from build123d import *

# Parameters (mm, degrees)
F0_W     = 106
F0_H     = 100
F0_R     = 2.706104
F0_R_2   = 5
F0_W_2   = 80
F0_H_2   = 52
F1_DEPTH = 31
F2_R     = 10
F3_DEPTH = 2.5
F4_W     = 48
F4_H     = 15
F5_DEPTH = 2.5
F6_W     = 4.25
F6_H     = 28.5
F7_DEPTH = 2.5


with BuildPart() as f1:
    # F0 (on Front) → F1 (new body)
    with BuildSketch(Plane.XZ):
        Rectangle(F0_W, F0_H)
        with Locations((0, -37.5)):
            Circle(F0_R, mode=Mode.SUBTRACT)
        with Locations((16.9, -34.7)):
            Circle(F0_R_2, mode=Mode.SUBTRACT)
        with Locations((32.5, -37.5)):
            Circle(F0_R, mode=Mode.SUBTRACT)
        with Locations((0, 10.5)):
            Rectangle(F0_W_2, F0_H_2, mode=Mode.SUBTRACT)
        with Locations((0, 10.5)):
            Rectangle(F0_W_2, F0_H_2)
        with Locations((0, -37.5)):
            Circle(F0_R)
        with Locations((16.9, -34.7)):
            Circle(F0_R_2)
        with Locations((32.5, -37.5)):
            Circle(F0_R)
    extrude(amount=-F1_DEPTH)

    # F2
    f2_edges = [f1.edges().sort_by_distance(p)[0] for p in [
        (53, 15.5, -50),
        (53, 15.5, 50),
        (-53, 15.5, 50),
        (-53, 15.5, -50),
    ]]
    fillet(f2_edges, radius=F2_R)

    # F0 (on Front) → F3 (cut)
    with BuildSketch(Plane.XZ):
        with Locations((0, 10.5)):
            Rectangle(F0_W_2, F0_H_2)
        with Locations((0, -37.5)):
            Circle(F0_R)
        with Locations((16.9, -34.7)):
            Circle(F0_R_2)
        with Locations((32.5, -37.5)):
            Circle(F0_R)
    extrude(amount=-F3_DEPTH, mode=Mode.SUBTRACT)

    # F4 (on face) → F5 (cut)
    with BuildSketch(Plane(origin=(0, 31, 0), x_dir=(-1, 0, 0), z_dir=(0, 1, 0))):
        with Locations((19, 10)):
            Rectangle(F4_W, F4_H)
    extrude(amount=-F5_DEPTH, mode=Mode.SUBTRACT)

    # F6 (on face) → F7 (cut)
    with BuildSketch(Plane.YZ.offset(53)):
        with Locations((16.375, -4)):
            Rectangle(F6_W, F6_H)
    extrude(amount=-F7_DEPTH, mode=Mode.SUBTRACT)


solid = f1.part
For this review, take the finished solid that the model builds, in its own axes (mm). A direction names the side the tool comes from. Round coordinates to 2 decimals unless told otherwise and drop trailing zeros. Write each loop counter-clockwise with the first axis right and the second up, starting at its lowest first coordinate (ties: lowest second). Pieces come first, ordered by that corner, then holes. Notation, with made-up numbers: (76.5, 4.25) - (132.5, 4.25) arc R27 ccw to (132.5, 35.25) - close; hole circle Ø9 at (61.25, -16.75). An arc over 180 degrees is marked (long way). Use a Markdown table: item, result.
Q1. We need section B-B (z = 25). Give the boundary of the cut face in (x, y).
Derived:
| item | result |
|---|---|
| outline | (-53, 0) - (-40, 0) - (-40, 2.5) - (40, 2.5) - (40, 0) - (53, 0) - (53, 31) - (-53, 31) - close |
Q2. We need section C-C (x = 16.9). Give the boundary of the cut face in (y, z).
Derived:
| item | result |
|---|---|
| outline | (0, -50) - (31, -50) - (31, 50) - (0, 50) - (0, 36.5) - (2.5, 36.5) - (2.5, -15.5) - (0, -15.5) - (0, -29.7) - (2.5, -29.7) - (2.5, -39.7) - (0, -39.7) - close |
Q3. Machinability: for faces 1 (the flat face through (-19, 30, 2.5)), 2 (the flat face through (52, 18.5, -4)), 3 (the cylindrical face through (35, 1.23, -38.54)), which of the approach directions +Z, -Z, +X, -X, +Y, -Y give a long, thin tool a straight path to every point of the face, cutting with its end or side? Answer none if there is none.
Derived:
| item | result |
|---|---|
| face 1 | +Y |
| face 2 | +X |
| face 3 | -Y |
Q4. The part is to be moulded in two halves that separate along Z. For faces 4 (the flat face through (52, 16, 10.25)), 5 (the flat face through (-1, 31, 1)), 6 (the cylindrical face through (-50.15, 15.72, -46.99)), say which applies: pulls with the +Z half, pulls with the -Z half, needs draft (parallel to the pull), parting line crosses it, or undercut.
Derived:
| item | result |
|---|---|
| face 4 | undercut |
| face 5 | needs draft |
| face 6 | pulls with the -Z half |
Q5. We need section D-D (x = 0). Give the boundary of the cut face in (y, z).
Derived:
| item | result |
|---|---|
| outline | (0, -50) - (31, -50) - (31, 2.5) - (28.5, 2.5) - (28.5, 17.5) - (31, 17.5) - (31, 50) - (0, 50) - (0, 36.5) - (2.5, 36.5) - (2.5, -15.5) - (0, -15.5) - (0, -34.79) - (2.5, -34.79) - (2.5, -40.21) - (0, -40.21) - close |
Q6. Wall thickness on line 1 along Z through (x, y) = (16.9, 0.9); line 2 along Z through (x, y) = (0, 1.05); line 3 along Y through (x, z) = (1, -37.5): over which ranges is each line inside the solid? List them lowest first.
Derived:
| item | result |
|---|---|
| line 1 | z = -50 to -39.7, -29.7 to -15.5, 36.5 to 50 |
| line 2 | z = -50 to -40.21, -34.79 to -15.5, 36.5 to 50 |
| line 3 | y = 2.5 to 31 |
Q7. Clearance check with flat-ended pins moving along their axes: pin 1 (2 mm diameter, centred on x = 51.5, y = 15.5, fed in from -Z); pin 2 (3 mm diameter, centred on x = 0, z = -37.5, fed in from -Y); pin 3 (7.5 mm diameter, centred on x = -8, z = 8.5, fed in from +Y). State where each tip first meets the part, or that it passes through.
Derived:
| item | result |
|---|---|
| pin 1 | stops at z = -46.61 |
| pin 2 | stops at y = 2.5 |
| pin 3 | stops at y = 28.5 |
Q8. We need section A-A (x = 32.5). Give the boundary of the cut face in (y, z).
Derived:
| item | result |
|---|---|
| outline | (0, -50) - (31, -50) - (31, 50) - (0, 50) - (0, 36.5) - (2.5, 36.5) - (2.5, -15.5) - (0, -15.5) - (0, -34.79) - (2.5, -34.79) - (2.5, -40.21) - (0, -40.21) - close |
